Source: CAD feature listing. Evaluate the final solid. Frame: model axes, mm. Face numbers are marked on the shaded views. A direction names the side the tool comes from. Give positions to 0.01 mm unless a question says otherwise; leave off trailing zeros. Order: outer loops, then holes, each group sorted by start corner. A loop starts at its lowest first (then second) coordinate and runs counter-clockwise, first axis right, second up. Notation, with made-up numbers: (0, -22) - (41, -22) arc R21 cw to (41, -13) - close; hole circle Ø4 at (5, -23.75). An arc over 180 degrees is marked (long way). Write each question's results on one line, items separated by ' | '. Start each with the question number.
Item 1: Section B-B on x = 0. Output: boundary loops of the cut face in (y, z).
Item 2: Section C-C on z = 55. Output: boundary loops of the cut face in (x, y).
Item 3: Section A-A on y = 0. Output: boundary loops of the cut face in (x, z), and give its area (3 significant figures).
Item 4: Section D-D on y = 5. Output: boundary loops of the cut face in (x, z), and give its area (3 significant figures).
Item 5: Contact query for flat-ended pins moving along their axis: pin 1 Ø3.5 at (x, y) = (-14, -7.5) entering from -Z; pin 2 Ø12 at (y, z) = (9.5, 33) entering from -X; pin 3 Ø1.9 at (x, y) = (13.42, -7.75) entering from +Z. Output: stop coordinate, or through.
Item 6: Line query: line 1 along Y through (x, z) = (0, 3); line 2 along X through (y, z) = (-7.75, 6.5); line 3 along Y through (x, z) = (-12, 4.5). Output: solid intervals per line, ascending.
Item 7: Set-up query: the marked faces 1 and 2. Return all of +Z, -Z, +X, -X, +Y, -Y with unobstructed straight access to the full face (end or side cutting, diameter ignored); none if empty.
Item 8: Mould query, pull axis Z, two halves, no side actions, for the marked faces 3, 4 and 5. Classes: released by +Z, released by -Z, zero draft, split by the parting line, or undercut.
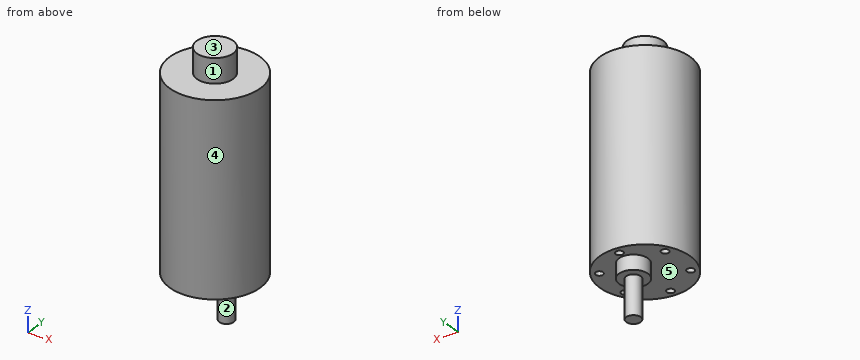
```python
from build123d import *

# Parameters (mm, degrees)
SKETCH_1_R               = 18.7
EXTRUDE_1_DEPTH          = 78
SKETCH_2_R               = 7.5
EXTRUDE_2_DEPTH          = 10
CUT_EXTRUDE_1_DEPTH      = 92.887866446
CUT_EXTRUDE_1_DEPTH_BACK = 10
SKETCH_3_R               = 1.55
SKETCH_4_R               = 6
EXTRUDE_3_DEPTH          = 6
SKETCH_5_R               = 3
EXTRUDE_4_DEPTH          = 16


with BuildPart() as part:
    # 草图1 → 凸台-拉伸1 (new body)
    with BuildSketch(Plane.XY):
        Circle(SKETCH_1_R)
    extrude(amount=EXTRUDE_1_DEPTH)

    # 草图2 → 凸台-拉伸2 (add)
    with BuildSketch(Plane.XY.offset(78)):
        Circle(SKETCH_2_R)
    extrude(amount=EXTRUDE_2_DEPTH)

    # 草图3 → 切除-拉伸1 (cut, two sides: drawn at the far end of the back side and taken through both)
    with BuildSketch(Plane(origin=(0, 0, 0), x_dir=(-1, 0, 0), z_dir=(0, 0, -1)).offset(-CUT_EXTRUDE_1_DEPTH_BACK)):
        with Locations(Location((0, 15.5, 0), (0, 0, 180))):
            Circle(SKETCH_3_R)
        with Locations(Location((13.423393759, 7.75, 0), (0, 0, 180))):
            Circle(SKETCH_3_R)
        with Locations(Location((13.423393759, -7.75, 0), (0, 0, 180))):
            Circle(SKETCH_3_R)
        with Locations(Location((0, -15.5, 0), (0, 0, 180))):
            Circle(SKETCH_3_R)
        with Locations(Location((-13.423393759, -7.75, 0), (0, 0, 180))):
            Circle(SKETCH_3_R)
        with Locations(Location((-13.423393759, 7.75, 0), (0, 0, 180))):
            Circle(SKETCH_3_R)
    extrude(amount=CUT_EXTRUDE_1_DEPTH + CUT_EXTRUDE_1_DEPTH_BACK, mode=Mode.SUBTRACT)

    # 草图4 → 凸台-拉伸3 (add)
    with BuildSketch(Plane(origin=(0, 0, 0), x_dir=(-1, 0, 0), z_dir=(0, 0, -1))):
        with Locations(Location((0, 7, 0), (0, 0, 180))):
            Circle(SKETCH_4_R)
    extrude(amount=EXTRUDE_3_DEPTH)

    # 草图5 → 凸台-拉伸4 (add)
    with BuildSketch(Plane(origin=(0, 0, -6), x_dir=(-1, 0, 0), z_dir=(0, 0, -1))):
        with Locations((0, 7)):
            Circle(SKETCH_5_R)
    extrude(amount=EXTRUDE_4_DEPTH)


solid = part.part
```
Evaluation:
1) outline: (-18.7, 0) - (-17.05, 0) - (-17.05, 10) - (-13.95, 10) - (-13.95, 0) - (1, 0) - (1, -6) - (4, -6) - (4, -22) - (10, -22) - (10, -6) - (13, -6) - (13, 0) - (13.95, 0) - (13.95, 10) - (17.05, 10) - (17.05, 0) - (18.7, 0) - (18.7, 78) - (7.5, 78) - (7.5, 88) - (-7.5, 88) - (-7.5, 78) - (-18.7, 78) - close
2) outline: circle Ø37.4 at (0, 0)
3) outline: (-18.7, 0) - (18.7, 0) - (18.7, 78) - (7.5, 78) - (7.5, 88) - (-7.5, 88) - (-7.5, 78) - (-18.7, 78) - close | area: 3,070 mm^2
4) outline: (-18.02, 0) - (-5.66, 0) - (-5.66, -6) - (-2.24, -6) - (-2.24, -22) - (2.24, -22) - (2.24, -6) - (5.66, -6) - (5.66, 0) - (18.02, 0) - (18.02, 78) - (5.59, 78) - (5.59, 88) - (-5.59, 88) - (-5.59, 78) - (-18.02, 78) - close | area: 3,060 mm^2
5) pin 1: stops at z = 0 | pin 2: stops at x = -18.37 | pin 3: stops at z = 78
6) line 1: y = -18.7 to -17.05, -13.95 to 13.95, 17.05 to 18.7 | line 2: x = -17.02 to -14.97, -11.87 to 11.87, 14.97 to 17.02 | line 3: y = -14.34 to -8.36, -7.14 to 7.14, 8.36 to 14.34
7) face 1: +Z | face 2: -Z
8) face 3: released by +Z | face 4: zero draft | face 5: released by -Z
